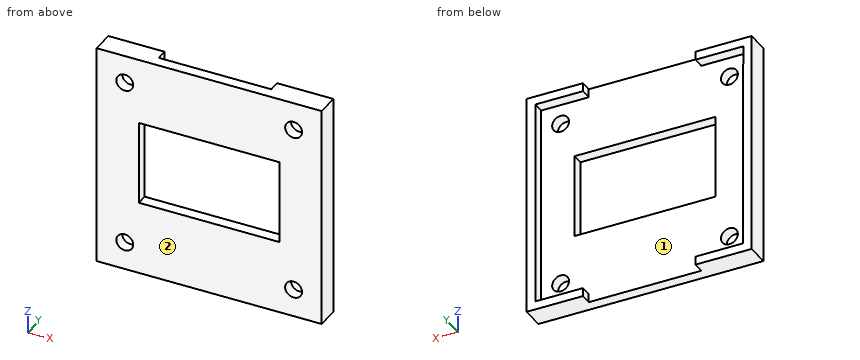
from build123d import *

# Parameters (mm, degrees)
SKETCH1_W           = 40
SKETCH1_H           = 40
SKETCH1_R           = 1.5
BOSS_EXTRUDE1_DEPTH = 2
BOSS_EXTRUDE2_DEPTH = 2
SKETCH3_W           = 25
SKETCH3_H           = 15
CUT_EXTRUDE1_DEPTH  = 2


with BuildPart() as part:
    # Sketch1 → Boss-Extrude1 (new body)
    with BuildSketch(Plane(origin=(0, 0, 0), x_dir=(1, 0, 0), z_dir=(0, 1, 0))):
        with Locations((0, 0.674157303)):
            Rectangle(SKETCH1_W, SKETCH1_H)
        with Locations(Location((-15, 15.674157303, 0), (0, 0, 270))):
            Circle(SKETCH1_R, mode=Mode.SUBTRACT)
        with Locations(Location((15, 15.674157303, 0), (0, 0, 270))):
            Circle(SKETCH1_R, mode=Mode.SUBTRACT)
        with Locations(Location((15, -14.325842697, 0), (0, 0, 90))):
            Circle(SKETCH1_R, mode=Mode.SUBTRACT)
        with Locations(Location((-15, -14.325842697, 0), (0, 0, 90))):
            Circle(SKETCH1_R, mode=Mode.SUBTRACT)
    extrude(amount=BOSS_EXTRUDE1_DEPTH)

    # Sketch2 → Boss-Extrude2 (add)
    with BuildSketch(Plane(origin=(0, 2, 0), x_dir=(1, 0, 0), z_dir=(0, 1, 0))):
        Polygon((-10, 19.174157303), (-10, 20.674157303), (-20, 20.674157303), (-20, -19.325842697), (-10, -19.325842697), (-10, -17.825842697), (-18.447674419, -17.825842697), (-18.499771919, -17.825842697), (-18.447674419, 19.174157303), align=None)
        Polygon((10, -19.325842697), (10, -17.825842697), (18.447674419, -17.825842697), (18.447674419, 19.174157303), (10, 19.174157303), (10, 20.674157303), (20, 20.674157303), (20, -19.325842697), align=None)
    extrude(amount=BOSS_EXTRUDE2_DEPTH)

    # Sketch3 → Cut-Extrude1 (cut)
    with BuildSketch(Plane.XZ):
        Rectangle(SKETCH3_W, SKETCH3_H)
    extrude(amount=-CUT_EXTRUDE1_DEPTH, mode=Mode.SUBTRACT)


solid = part.part
Verification items for the finished model (mm, model axes). Face numbers are marked on the shaded views. Coordinates: 2 decimals unless noted, no trailing zeros. Write each loop counter-clockwise with the first axis right and the second up, starting at its lowest first coordinate (ties: lowest second). Pieces come first, ordered by that corner, then holes. Notation, with made-up numbers: (88, -5) - (105, -5) arc R20 cw to (105, 16) - close; hole circle Ø2 at (17, 0). An arc over 180 degrees is marked (long way). Answer as a JSON object with one key per item and string values.
(1) Gauge pin test, flat end, axial feed: pin 1 Ø11 at (x, z) = (5, 8) entering from +Y. Record the tip position at first contact, or that the pin passes through.
Report:
{"pin 1": "y = 2"}
(2) Cross-section at A-A on y = 0.5. Record the cut outline in (x, z), plus the area to 3 significant figures.
Report:
{"outline": "(-20, -20.67) - (20, -20.67) - (20, 19.33) - (-20, 19.33) - close; hole circle Ø3 at (-15, -15.67); hole circle Ø3 at (-15, 14.33); hole (-12.5, -7.5) - (12.5, -7.5) - (12.5, 7.5) - (-12.5, 7.5) - close; hole circle Ø3 at (15, -15.67); hole circle Ø3 at (15, 14.33)", "area": "1,200 mm^2"}
(3) Thickness scan on line 1 along Z through (x, y) = (-11, 2.3); line 2 along X through (y, z) = (1.85, 15.5); line 3 along X through (y, z) = (3.25, 9.5). Record the ranges inside material, lowest first.
Report:
{"line 1": "-20.67 to -19.17, 17.83 to 19.33", "line 2": "-20 to -15.93, -14.07 to 14.07, 15.93 to 20", "line 3": "-20 to -18.49, 18.45 to 20"}
(4) Cross-section at B-B on x = 9.5. Record the cut outline in (y, z).
Report:
{"outline": "(0, -20.67) - (2, -20.67) - (2, -7.5) - (0, -7.5) - close; (0, 7.5) - (2, 7.5) - (2, 19.33) - (0, 19.33) - close"}
(5) Mould release check, pull along Z, two halves, no side actions. Record for the marked faces 1 and 2: pulls with the +Z half, pulls with the -Z half, needs draft (parallel to the pull), parting line crosses it, or undercut.
Report:
{"face 1": "undercut", "face 2": "needs draft"}
(6) Cross-section at D-D on z = -1. Record the cut outline in (x, y).
Report:
{"outline": "(-20, 0) - (-12.5, 0) - (-12.5, 2) - (-18.47, 2) - (-18.47, 4) - (-20, 4) - close; (12.5, 0) - (20, 0) - (20, 4) - (18.45, 4) - (18.45, 2) - (12.5, 2) - close"}
(7) Cross-section at C-C on x = 15. Record the cut outline in (y, z).
Report:
{"outline": "(0, -20.67) - (4, -20.67) - (4, -19.17) - (2, -19.17) - (2, -17.17) - (0, -17.17) - close; (0, -14.17) - (2, -14.17) - (2, 12.83) - (0, 12.83) - close; (0, 15.83) - (2, 15.83) - (2, 17.83) - (4, 17.83) - (4, 19.33) - (0, 19.33) - close"}
